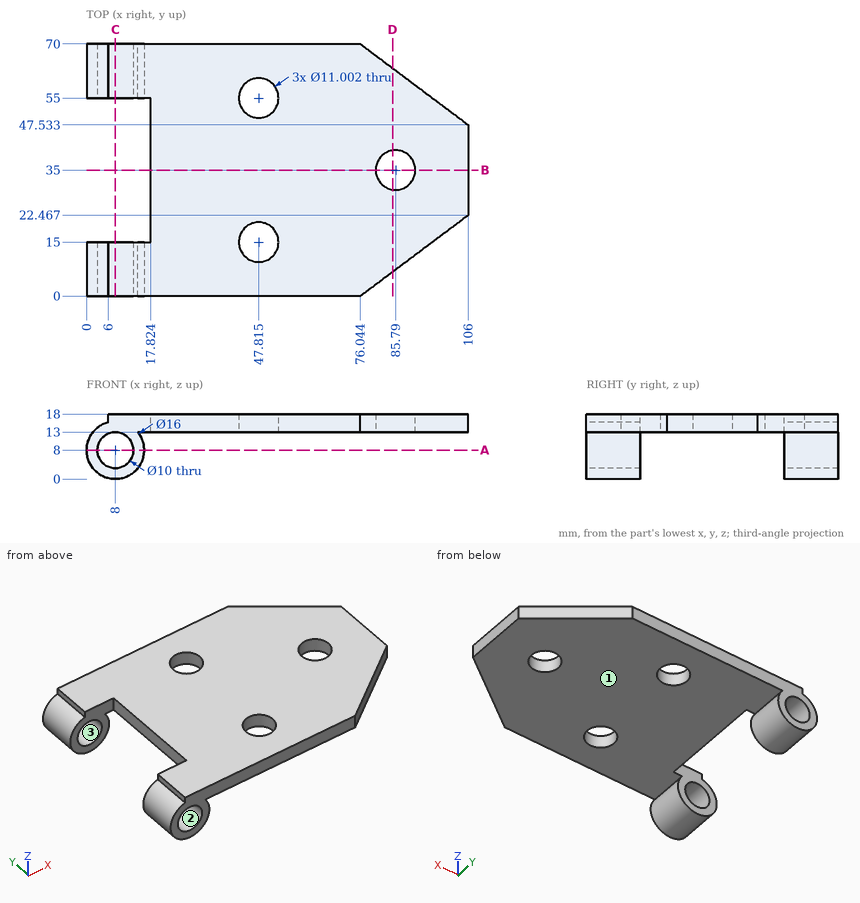
Here's the drawing with two shaded views (mm, measured from the low corner). I have some questions. Give positions to 0.01 mm unless a question says otherwise; leave off trailing zeros. Order: outer loops, then holes, each group sorted by start corner. A loop starts at its lowest first (then second) coordinate and runs counter-clockwise, first axis right, second up. Notation, with made-up numbers: M 67,15 L 74,15 A9 ccw 74,29 Z; hole C 40,19.25 d3. An arc over 180 degrees is marked long. One line per item, written item: value.
1) For P1, Ø9, axis at x = 8, z = 8, coming from the -Y side; P2, Ø2.5, axis at y = 45, z = 15.5, coming from the -X side; P3, Ø5, axis at y = 60.5, z = 7.5, coming from the +X side; P4, Ø1.8, axis at y = 63, z = 17, coming from the -X side, each with a flat end and sliding along its axis, tell me the tip position at first contact or that it passes through.
Answer sheet:
P1: passes through
P2: stops at x = 17.82
P3: stops at x = 16
P4: stops at x = 6
2) I want a section at A-A, the plane z = 8. List the corners of the cut face in (x, y) for me, plus the area to 3 significant figures.
Answer sheet:
outline: M 0,0 L 3,0 L 3,15 L 0,15 Z; M 0,55 L 3,55 L 3,70 L 0,70 Z; M 13,0 L 16,0 L 16,15 L 13,15 Z; M 13,55 L 16,55 L 16,70 L 13,70 Z
area: 180 mm^2
3) I want a section at B-B, the plane y = 35. List the corners of the cut face in (x, z) for me, plus the area to 3 significant figures.
Answer sheet:
outline: M 17.82,13 L 80.29,13 L 80.29,18 L 17.82,18 Z; M 91.29,13 L 106,13 L 106,18 L 91.29,18 Z
area: 386 mm^2
4) I want a section at C-C, the plane x = 8. List the corners of the cut face in (y, z) for me.
Answer sheet:
outline: M 0,0 L 15,0 L 15,3 L 0,3 Z; M 0,13 L 15,13 L 15,18 L 0,18 Z; M 55,0 L 70,0 L 70,3 L 55,3 Z; M 55,13 L 70,13 L 70,18 L 55,18 Z
5) I want a section at D-D, the plane x = 85. List the corners of the cut face in (y, z) for me (1 decimal).
Answer sheet:
outline: M 6.7,13 L 29.6,13 L 29.6,18 L 6.7,18 Z; M 40.4,13 L 63.3,13 L 63.3,18 L 40.4,18 Z
6) Please list where these lines run through material, in increasing order: line 1 along Y through (x, z) = (48, 14.75); line 2 along Y through (x, z) = (11.5, 17); line 3 along X through (y, z) = (6, 8).
Answer sheet:
line 1: y = 0 to 9.5, 20.5 to 49.5, 60.5 to 70
line 2: y = 0 to 15, 55 to 70
line 3: x = 0 to 3, 13 to 16
7) We'd pull the mould along X, two halves only. Please class the marked faces 1, 2 and 3: released by +X, released by -X, zero draft, split by the parting line, or undercut.
Answer sheet:
face 1: zero draft
face 2: undercut
face 3: undercut
